Model file for the job. Use its own axes, mm. Coordinates: 2 decimals unless noted, no trailing zeros. Loops run counter-clockwise (first coordinate to the right, second up) from the corner with the lowest first, then second, coordinate; pieces in that order, holes last.
Autodesk Fusion 360 part; units mm, degrees
sketch "Sketch1" plane through (0, 0, 0) normal (0, 0, 1) x (1, 0, 0)
  line L0 (24, -15.05) -> (-24, -15.05)
  line L1 (-24, -15.05) -> (-24, 15.05)
  line L2 (-24, 15.05) -> (24, 15.05)
  line L3 (24, 15.05) -> (24, -15.05)
  line L4 (24, -15.05) -> (-24, 15.05) construction
  line L5 (-24, -15.05) -> (24, 15.05) construction
  line L6 (24, -15.05) -> (18.3, -15.05)
  line L7 (18.3, -15.05) -> (18.3, -8.95)
  line L8 (18.3, -8.95) -> (24, -8.95)
  line L9 (-24, -15.05) -> (-18.3, -15.05)
  line L10 (-18.3, -15.05) -> (-18.3, -8.95)
  line L11 (-18.3, -8.95) -> (-24, -8.95)
  line L12 (-18.3, -15.05) -> (0.7, -15.05)
  line L13 (18.3, -15.05) -> (2.5, -15.05)
  line L14 (2.5, -15.05) -> (2.5, -8.65)
  line L15 (2.5, -8.65) -> (0.7, -8.65)
  line L16 (0.7, -8.65) -> (0.7, -15.05)
  dimension "d1" = 48
  dimension "d2" = 30.1
  dimension "d3" = 5.7
  dimension "d4" = 6.1
  dimension "d5" = 5.7
  dimension "d6" = 6.1
  dimension "d7" = 19
  dimension "d8" = 15.8
  dimension "d9" = 6.4
extrude "Extrude1" add sketch "Sketch1" along normal blind 1.6 contours L0 L1 L2 L3 L7 L8 L10 L11 L12 L13 L14 L15 L16
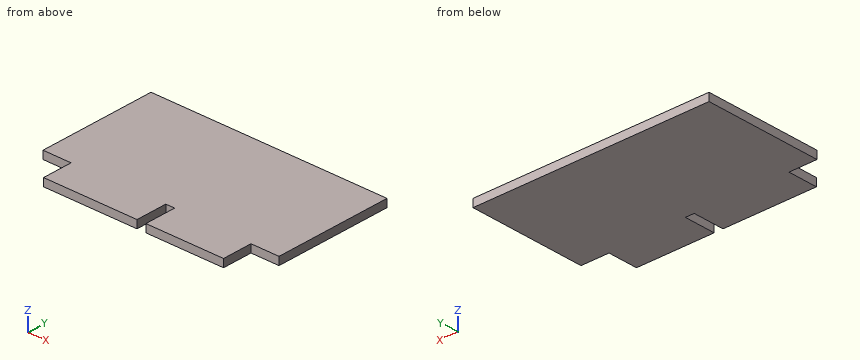
Q1. Drill centre lines: line 1 (X direction, y = -11, z = 1.4); line 2 (Y direction, x = 21.5, z = 0.9). Where is each one in solid material? Low to high.
Answers:
line 1: x = -18.3 to 0.7, 2.5 to 18.3
line 2: y = -8.95 to 15.05
Q2. Flat gauge pins, fed straight in: P1, Ø0.8, axis at y = -11, z = 1, coming from the -X side; P2, Ø0.5, axis at x = 2, z = 1, coming from the -Y side. Where does each tip first touch, or does it go through?
Answers:
P1: stops at x = -18.3
P2: stops at y = -8.65
Q3. Slice it at B-B (y = -12). List the corners of the cut face in (x, z), and give its area (3 significant figures).
Answers:
outline: (-18.3, 0) - (0.7, 0) - (0.7, 1.6) - (-18.3, 1.6) - close; (2.5, 0) - (18.3, 0) - (18.3, 1.6) - (2.5, 1.6) - close
area: 55.7 mm2
Q4. Slice it at C-C (x = -20). List the corners of the cut face in (y, z), and give its area (3 significant figures).
Answers:
outline: (-8.95, 0) - (15.05, 0) - (15.05, 1.6) - (-8.95, 1.6) - close
area: 38.4 mm2
Q5. Slice it at A-A (z = 0.7). List the corners of the cut face in (x, y), and give its area (3 significant figures).
Answers:
outline: (-24, -8.95) - (-18.3, -8.95) - (-18.3, -15.05) - (0.7, -15.05) - (0.7, -8.65) - (2.5, -8.65) - (2.5, -15.05) - (18.3, -15.05) - (18.3, -8.95) - (24, -8.95) - (24, 15.05) - (-24, 15.05) - close
area: 1,360 mm2
